Check sheet for the drawn part. Datum: minimum x, y, z corner. Units: mm. Coordinates: 2 decimals unless noted, no trailing zeros. Order: outer loops, then holes, each group sorted by start corner. A loop starts at its lowest first (then second) coordinate and runs counter-clockwise, first axis right, second up. Notation, with made-up numbers: M 33,44 L 39,44 A28 ccw 39,81 Z; hole C 41.5,24.25 d9. An arc over 180 degrees is marked long. Return JSON: item names as keys, results as strings. Group by question number.
Q1. Section check A-A, the plane y = 2.3. Count the separate pieces of the cut face and the enclosed holes in it, then the cut area to 3 significant figures.
Q2. Thickness scan on probe 1 along X at (y, z) = (2.85, 40) (1 decimal); probe 2 along X at (y, z) = (3.6, 16.5); probe 3 along Z at (x, y) = (38, 0.5). Record the ranges inside material, lowest first.
Q3. Section check D-D, the plane x = 31.5. Enter the section's corners in (y, z) (1 decimal), then the cut area to 3 significant figures.
Q4. Go/stop test with flat-tipped pins: pin 1 Ø2 at (y, z) = (0.5, 33.5) entering from -X; pin 2 Ø1.5 at (x, z) = (9.5, 32.5) entering from -Y; pin 3 Ø5.5 at (x, z) = (30, 5.43) entering from +Y. Record where each tip stops, or that it passes through.
Q5. Section check B-B, the plane x = 19. Enter the section's corners in (y, z).
Q6. Section check C-C, the plane z = 20. Enter the section's corners in (x, y).
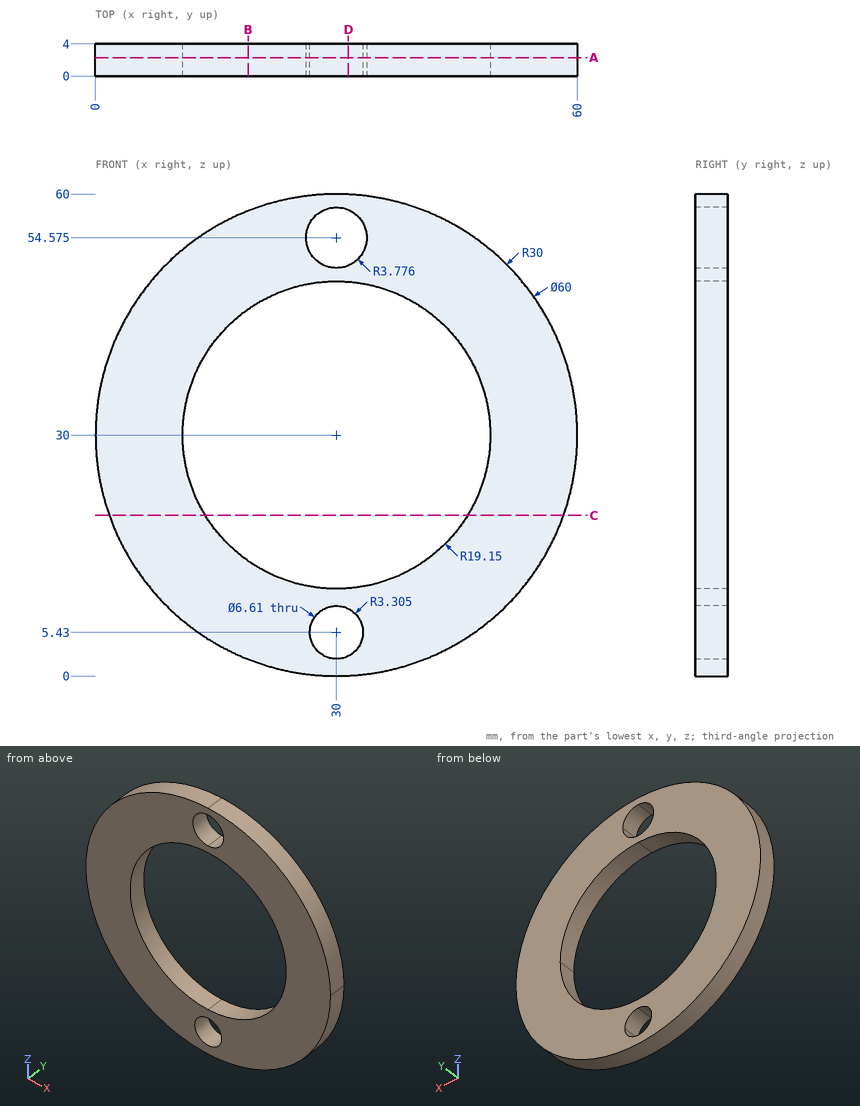
Numbers:
{
 "1": {"separate pieces": "1", "enclosed holes": "3", "area": "1,600 mm2"},
 "2": {"probe 1": "x = 1.7 to 13.7, 46.3 to 58.3", "probe 2": "x = 3.21 to 16.42, 43.58 to 56.79", "probe 3": "z = 1.09 to 12.6, 47.4 to 58.91"},
 "3": {"outline": "M 0,0 L 4,0 L 4,2.5 L 0,2.5 Z; M 0,8.4 L 4,8.4 L 4,10.9 L 0,10.9 Z; M 0,49.1 L 4,49.1 L 4,51.1 L 0,51.1 Z; M 0,58 L 4,58 L 4,60 L 0,60 Z", "area": "35.7 mm2"},
 "4": {"pin 1": "stops at x = 0.1", "pin 2": "stops at y = 0", "pin 3": "passes through"},
 "5": {"outline": "M 0,2.09 L 4,2.09 L 4,14.32 L 0,14.32 Z; M 0,45.68 L 4,45.68 L 4,57.91 L 0,57.91 Z"},
 "6": {"outline": "M 1.72,0 L 13.67,0 L 13.67,4 L 1.72,4 Z; M 46.33,0 L 58.28,0 L 58.28,4 L 46.33,4 Z"}
}
